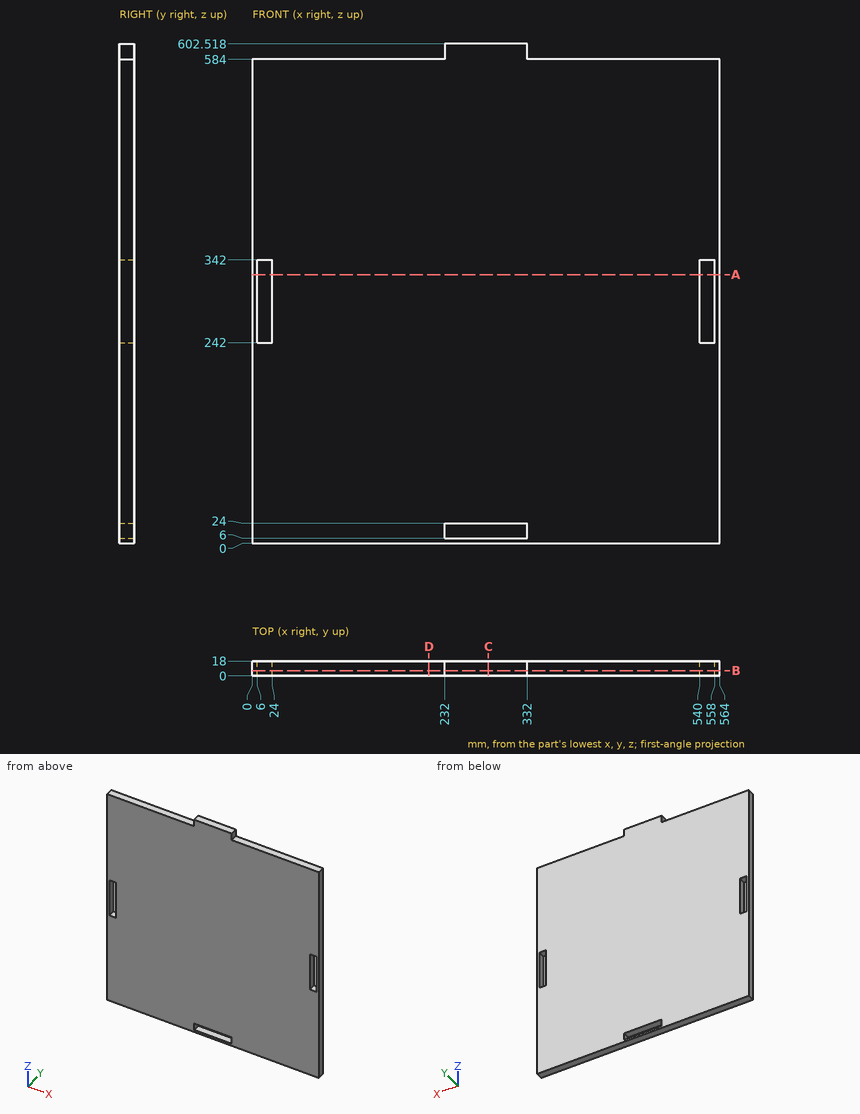
Print and shaded views of the part. All mm, measured from the part's lowest x, y and z. Coordinates: 2 decimals unless noted, no trailing zeros. Loops run counter-clockwise (first coordinate to the right, second up) from the corner with the lowest first, then second, coordinate; pieces in that order, holes last. Notation, with made-up numbers: (19.25, -22) - (71.25, -22) arc R26 cw to (71.25, 16) - close; hole circle Ø3 at (-15, -19.5). An arc over 180 degrees is marked (long way). Write item = value, one per line. Start each with the question number.
Item 1: Drop flat-ended pins along their axis: pin 1 Ø5.5 at (x, y) = (14, 8.5) entering from +Z; pin 2 Ø9 at (y, z) = (13.5, 595.5) entering from -X. Give the stop position or say it passes through.
Item 2: Saw through at A-A, the plane z = 324. List the corners of the cut face in (x, y), then the cut area to 3 significant figures.
Item 3: Saw through at B-B, the plane y = 6.5. List the corners of the cut face in (x, z).
Item 4: Wall check: probe 1 along X at (y, z) = (6.5, 311); probe 2 along Z at (x, y) = (319, 5.75); probe 3 along Z at (x, y) = (517.5, 9). Give the ranges that are in metal, low to high. Write a range as [from, to].
Item 5: Saw through at D-D, the plane x = 213. List the corners of the cut face in (y, z), then the cut area to 3 significant figures.
Item 6: Saw through at C-C, the plane x = 285. List the corners of the cut face in (y, z), then the cut area to 3 significant figures.
Answers:
q1.pin_1 = 584
q1.pin_2 = 232
q2.outline = (0, 0) - (6, 0) - (6, 18) - (0, 18) - close; (24, 0) - (540, 0) - (540, 18) - (24, 18) - close; (558, 0) - (564, 0) - (564, 18) - (558, 18) - close
q2.area = 9,500 mm2
q3.outline = (0, 0) - (564, 0) - (564, 584) - (332, 584) - (332, 602.52) - (232, 602.52) - (232, 584) - (0, 584) - close; hole (6, 242) - (24, 242) - (24, 342) - (6, 342) - close; hole (232, 6) - (332, 6) - (332, 24) - (232, 24) - close; hole (540, 242) - (558, 242) - (558, 342) - (540, 342) - close
q4.probe_1 = [0, 6], [24, 540], [558, 564]
q4.probe_2 = [0, 6], [24, 602.52]
q4.probe_3 = [0, 584]
q5.outline = (0, 0) - (18, 0) - (18, 584) - (0, 584) - close
q5.area = 10,500 mm2
q6.outline = (0, 0) - (18, 0) - (18, 6) - (0, 6) - close; (0, 24) - (18, 24) - (18, 602.52) - (0, 602.52) - close
q6.area = 10,500 mm2
